Build history of the part. All positions in model axes, mm. Face numbers are marked on the shaded views. Give positions to 0.01 mm unless a question says otherwise; leave off trailing zeros. Order: outer loops, then holes, each group sorted by start corner. A loop starts at its lowest first (then second) coordinate and runs counter-clockwise, first axis right, second up. Notation, with made-up numbers: (58, 11) - (64, 11) arc R27 ccw to (64, 47) - close; hole circle Ø3 at (77.5, -32). An arc over 180 degrees is marked (long way). Use a Markdown table: item, result. Add a question column.
(1) Mould opens along X. For the marked faces 1 and 2 say: +X half, -X half, draft (parallel to the pull), parting line (faces both ways), or undercut.
(2) Slice it at A-A (y = 0). Write the cut outline in (x, z).
(3) Slice it at B-B (y = -78.5). Write the cut outline in (x, z), then the cut area to 3 significant figures.
(4) Flat gauge pins, fed straight in: pin 1 (6.5 mm diameter, centred on x = -20, y = -30, fed in from +Z); pin 2 (3 mm diameter, centred on x = 29, z = 13.5, fed in from -Y); pin 3 (8 mm diameter, centred on x = -43, z = 7.5, fed in from -Y). Where does each tip first touch, or does it go through?
(5) Slice it at C-C (x = 45.5). Write the cut outline in (y, z).
(6) Wall check: line 1 (Y direction, x = -5, z = 6.25); line 2 (Y direction, x = 4, z = 8); line 3 (Y direction, x = 0, z = 1.45). Give the ranges that are in metal, low to high.
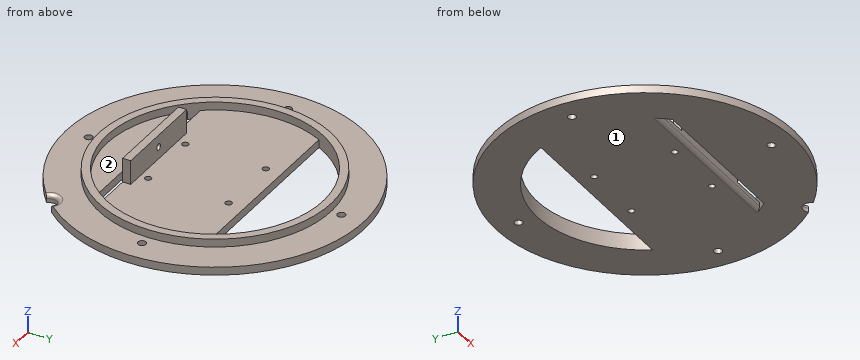
from build123d import *

# Parameters (mm, degrees)
SKETCH1_R           = 92.5
BOSS_EXTRUDE1_DEPTH = 5
SKETCH2_R           = 72
BOSS_EXTRUDE2_DEPTH = 5
SKETCH3_R           = 67
CUT_EXTRUDE1_DEPTH  = 11
SKETCH4_W           = 140
SKETCH4_H           = 70
BOSS_EXTRUDE3_DEPTH = 5
FILLET1_R           = 2.5
SKETCH7_W           = 110
SKETCH7_H           = 25
BOSS_EXTRUDE5_DEPTH = 5
SKETCH11_R          = 2
CUT_EXTRUDE4_DEPTH  = 5
SKETCH12_R          = 2.5
CUT_EXTRUDE5_DEPTH  = 5
SKETCH6_W           = 60
SKETCH6_H           = 5
BOSS_EXTRUDE6_DEPTH = 15
SKETCH13_R          = 2
CUT_EXTRUDE6_DEPTH  = 5
SKETCH14_R          = 5
CUT_EXTRUDE7_DEPTH  = 10
FILLET2_R           = 2.5


with BuildPart() as part:
    # Sketch1 → Boss-Extrude1 (new body)
    with BuildSketch(Plane.XY):
        Circle(SKETCH1_R)
    extrude(amount=BOSS_EXTRUDE1_DEPTH)

    # Sketch2 → Boss-Extrude2 (add)
    with BuildSketch(Plane.XY.offset(5)):
        Circle(SKETCH2_R)
    extrude(amount=BOSS_EXTRUDE2_DEPTH)

    # Sketch3 → Cut-Extrude1 (cut, through all)
    with BuildSketch(Plane(origin=(0, 0, 0), x_dir=(-1, 0, 0), z_dir=(0, 0, -1))):
        Circle(SKETCH3_R)
    extrude(amount=-CUT_EXTRUDE1_DEPTH, mode=Mode.SUBTRACT)

    # Sketch4 → Boss-Extrude3 (add)
    with BuildSketch(Plane(origin=(0, 0, 0), x_dir=(-1, 0, 0), z_dir=(0, 0, -1))):
        with Locations((0, -5)):
            Rectangle(SKETCH4_W, SKETCH4_H)
    extrude(amount=-BOSS_EXTRUDE3_DEPTH)

    # Fillet1
    fillet1_edges = [part.edges().sort_by_distance(p)[0] for p in [
        (0, -40, 0),
    ]]
    fillet(fillet1_edges, radius=FILLET1_R)

    # Sketch7 → Boss-Extrude5 (add)
    with BuildSketch(Plane(origin=(0, 0, 0), x_dir=(-1, 0, 0), z_dir=(0, 0, -1))):
        with Locations((0, -58)):
            Rectangle(SKETCH7_W, SKETCH7_H)
    extrude(amount=-BOSS_EXTRUDE5_DEPTH)

    # Sketch11 → Cut-Extrude4 (cut)
    with BuildSketch(Plane(origin=(0, 0, 0), x_dir=(-1, 0, 0), z_dir=(0, 0, -1))):
        with Locations((-20, -30)):
            Circle(SKETCH11_R)
        with Locations((-20, 20)):
            Circle(SKETCH11_R)
        with Locations((20, 20)):
            Circle(SKETCH11_R)
        with Locations((20, -30)):
            Circle(SKETCH11_R)
    extrude(amount=-CUT_EXTRUDE4_DEPTH, mode=Mode.SUBTRACT)

    # Sketch12 → Cut-Extrude5 (cut)
    with BuildSketch(Plane(origin=(0, 0, 0), x_dir=(-1, 0, 0), z_dir=(0, 0, -1))):
        with Locations((0, -78.5)):
            Circle(SKETCH12_R)
        with Locations((-78.5, 0)):
            Circle(SKETCH12_R)
        with Locations((0, 78.5)):
            Circle(SKETCH12_R)
        with Locations((78.5, 0)):
            Circle(SKETCH12_R)
    extrude(amount=-CUT_EXTRUDE5_DEPTH, mode=Mode.SUBTRACT)

    # Sketch6 → Boss-Extrude6 (add)
    with BuildSketch(Plane.XY.offset(5)):
        with Locations((0, -37.5)):
            Rectangle(SKETCH6_W, SKETCH6_H)
    extrude(amount=BOSS_EXTRUDE6_DEPTH)

    # Sketch13 → Cut-Extrude6 (cut)
    with BuildSketch(Plane.XZ.offset(40)):
        with Locations((0, 12.5)):
            Circle(SKETCH13_R)
    extrude(amount=-CUT_EXTRUDE6_DEPTH, mode=Mode.SUBTRACT)

    # Sketch14 → Cut-Extrude7 (cut)
    with BuildSketch(Plane(origin=(0, 0, 0), x_dir=(-1, 0, 0), z_dir=(0, 0, -1))):
        with Locations((-65.40737726, -65.40737726)):
            Circle(SKETCH14_R)
    extrude(amount=-CUT_EXTRUDE7_DEPTH, mode=Mode.SUBTRACT)

    # Fillet2
    fillet2_edges = [part.edges().sort_by_distance(p)[0] for p in [
        (61.871843354, -61.871843354, 5),
    ]]
    fillet(fillet2_edges, radius=FILLET2_R)


solid = part.part
Solution:
| question | item | result |
|---|---|---|
| 1 | face 1 | draft |
| 1 | face 2 | undercut |
| 2 | outline | (-92.5, 0) - (-81, 0) - (-81, 5) - (-92.5, 5) - close; (-76, 0) - (76, 0) - (76, 5) - (72, 5) - (72, 10) - (67, 10) - (67, 5) - (-67, 5) - (-67, 10) - (-72, 10) - (-72, 5) - (-76, 5) - close; (81, 0) - (92.5, 0) - (92.5, 5) - (81, 5) - close |
| 3 | outline | (-48.93, 0) - (-2.5, 0) - (-2.5, 5) - (-48.93, 5) - close; (2.5, 0) - (48.93, 0) - (48.93, 5) - (2.5, 5) - close |
| 3 | area | 464 mm2 |
| 4 | pin 1 | z = 5 |
| 4 | pin 2 | y = -40 |
| 4 | pin 3 | y = -83.46 |
| 5 | outline | (-80.54, 0) - (-45.5, 0) - (-45.5, 5) - (-49.18, 5) - (-49.18, 10) - (-55.8, 10) - (-55.8, 5) - (-80.54, 5) - close; (-40, 2.5) arc R2.5 ccw to (-37.5, 0) - (30, 0) - (30, 5) - (-40, 5) - close; (49.18, 0) - (80.54, 0) - (80.54, 5) - (55.8, 5) - (55.8, 10) - (49.18, 10) - close |
| 6 | line 1 | -71.83 to -66.81, -40 to -35, 66.81 to 71.83 |
| 6 | line 2 | -71.89 to -66.88, -40 to -35, 66.88 to 71.89 |
| 6 | line 3 | -92.5 to -81, -76 to -45.5, -39.77 to 30, 67 to 76, 81 to 92.5 |
